Verification items for this drawing (mm, ordinates from the low corner). Round coordinates to 2 decimals unless told otherwise and drop trailing zeros. Loops run counter-clockwise (first coordinate to the right, second up) from the corner with the lowest first, then second, coordinate; pieces in that order, holes last. Notation, with made-up numbers: M 11,62.25 L 51,62.25 A18 cw 51,80.25 Z; hole C -2.5,23 d5. An arc over 180 degrees is marked long. Answer as CSV lines item,"result".
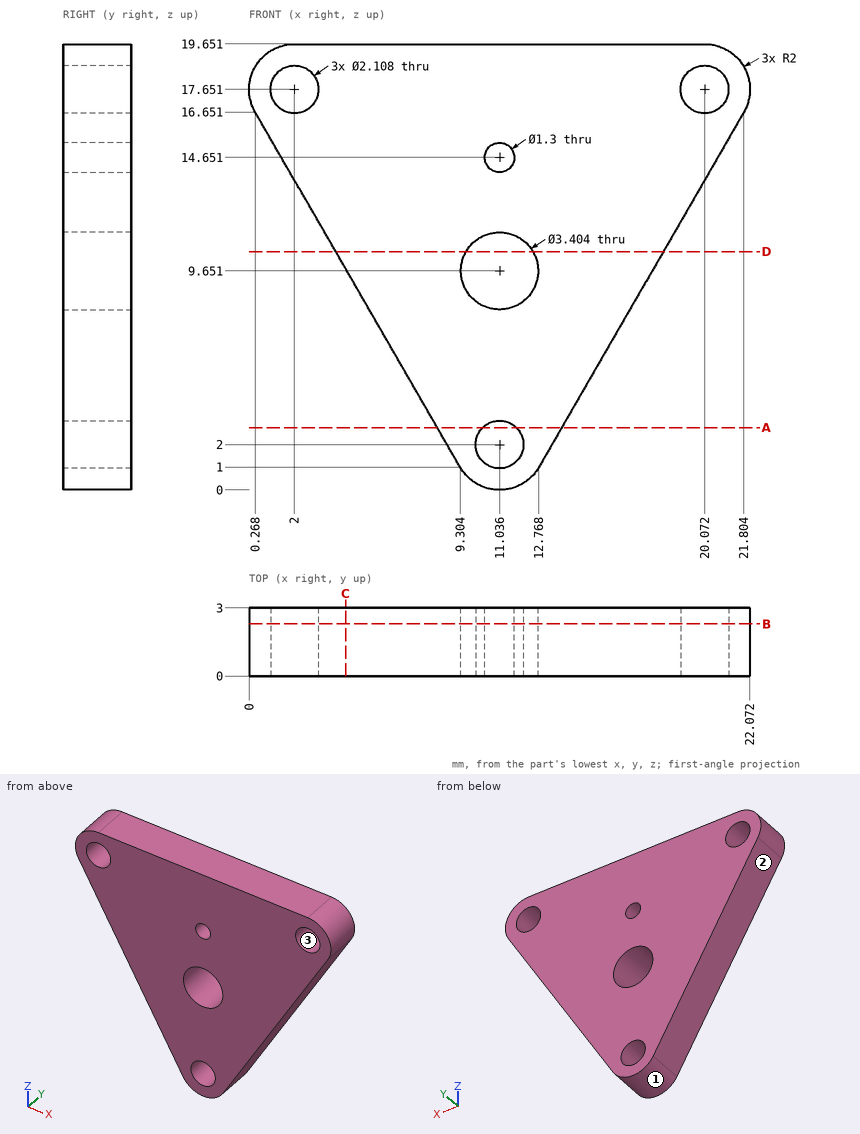
1) Material ranges on probe 1 along X at (y, z) = (0.85, 17.75); probe 2 along Z at (x, y) = (11, 0.85); probe 3 along X at (y, z) = (0.65, 8.75), recorded low to high.
Here are the results:
probe 1,"x = 0 to 0.95, 3.05 to 19.02, 21.12 to 22.07"
probe 2,"z = 0 to 0.95, 3.05 to 7.95, 11.35 to 14, 15.3 to 19.65"
probe 3,"x = 4.83 to 9.59, 12.48 to 17.24"
2) Go/stop test with a flat-tipped pin: pin 1 (1.5 mm diameter, centred on x = 10, y = 1, fed in from -Z). Record where the tip stops, or that it passes through.
Here are the results:
pin 1,"stops at z = 0.02"
3) Draft check along X on the marked faces 1, 2 and 3. Enter one of: +X half, -X half, draft (parallel to the pull), parting line (faces both ways), or undercut.
Here are the results:
face 1,"parting line"
face 2,"-X half"
face 3,"undercut"
4) Section check B-B (y = 2.3). State how many separate pieces and enclosed holes the cut face has.
Here are the results:
separate pieces,"1"
enclosed holes,"5"
5) Section check A-A (z = 2.75). Record the cut outline in (x, y) (1 decimal).
Here are the results:
outline,"M 8.3,0 L 10.3,0 L 10.3,3 L 8.3,3 Z; M 11.8,0 L 13.8,0 L 13.8,3 L 11.8,3 Z"
6) Section check D-D (z = 10.5). Record the cut outline in (x, y).
Here are the results:
outline,"M 3.82,0 L 9.56,0 L 9.56,3 L 3.82,3 Z; M 12.51,0 L 18.25,0 L 18.25,3 L 12.51,3 Z"
7) Section check C-C (x = 4.25). Record the cut outline in (y, z).
Here are the results:
outline,"M 0,9.75 L 3,9.75 L 3,19.65 L 0,19.65 Z"
